from build123d import *

# Parameters (mm, degrees)
SKETCH1_W           = 20
SKETCH1_H           = 6
BOSS_EXTRUDE1_DEPTH = 174.8
SKETCH2_W           = 20.4
SKETCH2_H           = 47.6
CUT_EXTRUDE1_DEPTH  = 2
SKETCH3_W           = 14
SKETCH3_H           = 14
BOSS_EXTRUDE2_DEPTH = 90
SKETCH4_W           = 0.3
SKETCH4_H           = 6
CUT_EXTRUDE2_DEPTH  = 175


with BuildPart() as part:
    # Sketch1 → Boss-Extrude1 (new body)
    with BuildSketch(Plane(origin=(0, 0, 0), x_dir=(1, 0, 0), z_dir=(0, 1, 0))):
        Rectangle(SKETCH1_W, SKETCH1_H)
    extrude(amount=BOSS_EXTRUDE1_DEPTH)

    # Sketch2 → Cut-Extrude1 (cut)
    with BuildSketch(Plane.XY.offset(3)):
        with Locations((10, 87.4)):
            Rectangle(SKETCH2_W, SKETCH2_H)
    extrude(amount=-CUT_EXTRUDE1_DEPTH, mode=Mode.SUBTRACT)

    # Sketch3 → Boss-Extrude2 (add)
    with BuildSketch(Plane(origin=(0, 0, -3), x_dir=(-1, 0, 0), z_dir=(0, 0, -1))):
        with Locations((3, 31.9)):
            Rectangle(SKETCH3_W, SKETCH3_H)
    boss_extrude2 = extrude(amount=BOSS_EXTRUDE2_DEPTH)

    # Mirror1: Boss-Extrude2 across plane
    add(boss_extrude2.mirror(Plane.ZX.offset(87.4)))

    # Sketch4 → Cut-Extrude2 (cut)
    with BuildSketch(Plane.XZ):
        with Locations((9.85, 0)):
            Rectangle(SKETCH4_W, SKETCH4_H)
    extrude(amount=-CUT_EXTRUDE2_DEPTH, mode=Mode.SUBTRACT)


solid = part.part
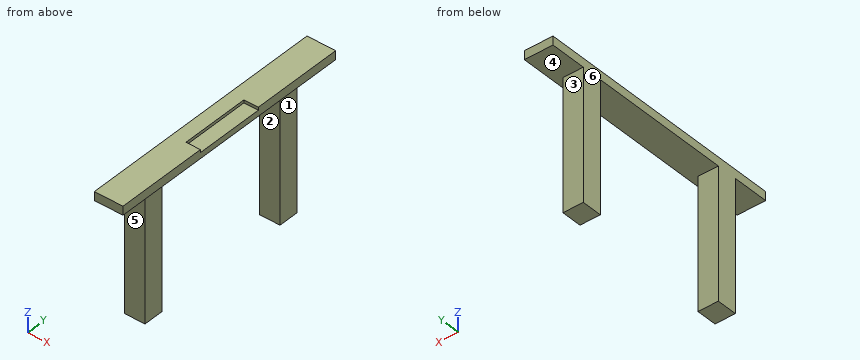
Verification items for the finished model (mm, model axes). Face numbers are marked on the shaded views. A direction names the side the tool comes from. Round coordinates to 2 decimals unless told otherwise and drop trailing zeros. Loops run counter-clockwise (first coordinate to the right, second up) from the corner with the lowest first, then second, coordinate; pieces in that order, holes last. Notation, with made-up numbers: M 61,-8 L 98,-8 A12 cw 98,1 Z; hole C 39.5,65.25 d5. An arc over 180 degrees is marked long. Write each question's results on one line, items separated by ' | '.
1) Mould release check, pull along Y, two halves, no side actions. Record for the marked faces 4, 5 and 6: released by +Y, released by -Y, zero draft, split by the parting line, or undercut.
Checks:
face 4: undercut | face 5: released by -Y | face 6: zero draft
2) Section check B-B on x = -7.5. Record the boundary of the cut face in (y, z).
Checks:
outline: M 0,-3 L 24.9,-3 L 24.9,-93 L 38.9,-93 L 38.9,-3 L 135.9,-3 L 135.9,-93 L 149.9,-93 L 149.9,-3 L 174.8,-3 L 174.8,3 L 0,3 Z
3) Gauge pin test, flat ends, axial feed: P1, Ø7, axis at x = -4.5, z = -29, coming from the -Y side; P2, Ø7, axis at y = 29, z = -29, coming from the +X side; P3, Ø5, axis at x = 5.5, z = -38, coming from the +Y side. Record the tip position at first contact, or that the pin passes through.
Checks:
P1: stops at y = 24.9 | P2: stops at x = 4 | P3: stops at y = 149.9
4) Section check A-A on z = -76.5. Record the boundary of the cut face in (x, y), then the cut area to 3 significant figures.
Checks:
outline: M -10,24.9 L 4,24.9 L 4,38.9 L -10,38.9 Z; M -10,135.9 L 4,135.9 L 4,149.9 L -10,149.9 Z | area: 392 mm2
5) Section check D-D on y = 34.5. Record the boundary of the cut face in (x, z).
Checks:
outline: M -10,-93 L 4,-93 L 4,-3 L 9.7,-3 L 9.7,3 L -10,3 Z
6) Access from +Z, -Z, +X, -X, +Y, -Y to the whole of each face (thin tool, end or side, straight path). Record for the marked faces 1, 2 and 3.
Checks:
face 1: -Z, +X, +Y, -Y | face 2: -Z, +X, -X | face 3: -Z, +X, -X, +Y
7) Scan lines: L1, parallel to Y at x = 0.25, z = -83.5; L2, parallel to Z at x = -2.25, y = 83; L3, parallel to X at y = 35, z = -9.5. Record each from-to range of solid material in increasing order. Write a range as from..to.
Checks:
L1: y = 24.9..38.9, 135.9..149.9 | L2: z = -3..3 | L3: x = -10..4
8) Section check C-C on y = 67.5. Record the boundary of the cut face in (x, z), then the cut area to 3 significant figures.
Checks:
outline: M -10,-3 L 9.7,-3 L 9.7,1 L -0.2,1 L -0.2,3 L -10,3 Z | area: 98.4 mm2
